```python
from build123d import *

# Parameters (mm, degrees)
F0_W     = 25.4
F0_H     = 25.4
F1_DEPTH = 25.4
F2_T     = -2.54
F3_R     = 0.6096
F4_DEPTH = 12.8016
F5_R     = 0.6096
F6_DEPTH = 13.208


with BuildPart() as f1:
    # F0 (on Front) → F1 (new body)
    with BuildSketch(Plane.XZ):
        Rectangle(F0_W, F0_H)
    extrude(amount=F1_DEPTH)

    # F2
    f2_openings = [f1.faces().sort_by_distance(p)[0] for p in [
        (0, -12.7, 12.7),
    ]]
    offset(amount=F2_T, openings=f2_openings)

    # F3 (on face) → F4 (cut)
    with BuildSketch(Plane.XY.offset(12.7)):
        with Locations((-10.955215, -23.901867)):
            Circle(F3_R)
    extrude(amount=-F4_DEPTH, mode=Mode.SUBTRACT)

    # F5 (on face) → F6 (cut)
    with BuildSketch(Plane.XY.offset(12.7)):
        with Locations((11.037277, -1.745251)):
            Circle(F5_R)
    extrude(amount=-F6_DEPTH, mode=Mode.SUBTRACT)


solid = f1.part
```
Work out the finished part from the listing and answer in its coordinate system (mm). A direction names the side the tool comes from. Give positions to 0.01 mm unless a question says otherwise; leave off trailing zeros. Write each loop counter-clockwise with the first axis right and the second up, starting at its lowest first coordinate (ties: lowest second). Pieces come first, ordered by that corner, then holes. Notation, with made-up numbers: (17.5, 86) - (70.5, 86) arc R27 ccw to (70.5, 121) - close; hole circle Ø9 at (47.5, 45.5). An arc over 180 degrees is marked (long way). Use one line per item in the form item = value.
1. Consider L1, parallel to Y at x = 4.5, z = -1; L2, parallel to X at y = -11, z = -8; L3, parallel to Z at x = -4.25, y = -2.75. Determine where each line is inside the solid, lowest interval first.
Filled in:
L1 = -25.4 to -22.86, -2.54 to 0
L2 = -12.7 to -10.16, 10.16 to 12.7
L3 = -12.7 to -10.16
2. A cutting plane is placed at D-D (z = 1.25). Write down the section's boundary in (x, y).
Filled in:
outline = (-12.7, -25.4) - (12.7, -25.4) - (12.7, 0) - (-12.7, 0) - close; hole circle Ø1.22 at (-10.96, -23.9); hole (-10.16, -22.86) - (10.16, -22.86) - (10.16, -2.54) - (-10.16, -2.54) - close; hole circle Ø1.22 at (11.04, -1.75)
3. Each of these flat-tipped pins is pushed along its axis until it touches: pin 1 Ø1 at (x, y) = (5, -20) entering from +Z; pin 2 Ø0.6 at (x, y) = (-11, -24) entering from +Z. Where does it stop, or does it pass through?
Filled in:
pin_1 = -10.16
pin_2 = -0.1
4. For faces 1 (the face through (-11, -24, -0.102)), 2 (the face through (0, -13, -12.7)), determine the directions among +Z, -Z, +X, -X, +Y, -Y from which every point of the face is accessible in a straight line to the end or side of a thin tool.
Filled in:
face_1 = +Z
face_2 = -Z, +X, -X, +Y, -Y
5. A cutting plane is placed at B-B (x = -5.25). Write down the section's boundary in (y, z), and give its area (3 significant figures).
Filled in:
outline = (-25.4, -12.7) - (0, -12.7) - (0, 12.7) - (-2.54, 12.7) - (-2.54, -10.16) - (-22.86, -10.16) - (-22.86, 12.7) - (-25.4, 12.7) - close
area = 181 mm^2
6. A cutting plane is placed at C-C (y = -8.75). Write down the section's boundary in (x, z).
Filled in:
outline = (-12.7, -12.7) - (12.7, -12.7) - (12.7, 12.7) - (10.16, 12.7) - (10.16, -10.16) - (-10.16, -10.16) - (-10.16, 12.7) - (-12.7, 12.7) - close
7. A cutting plane is placed at A-A (z = -5.5). Write down the section's boundary in (x, y), and give its area (3 significant figures).
Filled in:
outline = (-12.7, -25.4) - (12.7, -25.4) - (12.7, 0) - (-12.7, 0) - close; hole (-10.16, -22.86) - (10.16, -22.86) - (10.16, -2.54) - (-10.16, -2.54) - close
area = 232 mm^2
8. Determine the mould class of faces 3 (the face through (12.7, -13, 0)), 4 (the face through (10.16, -13, 1)), 5 (the face through (-12.7, -13, 0)) for opening direction X: released by +X, released by -X, zero draft, split by the parting line, or undercut.
Filled in:
face_3 = released by +X
face_4 = undercut
face_5 = released by -X
